The listing builds one solid part. Answer for the finished solid, in the listing's coordinates (mm). Face numbers are marked on the shaded views. A direction names the side the tool comes from. Give positions to 0.01 mm unless a question says otherwise; leave off trailing zeros. Order: outer loops, then holes, each group sorted by start corner. A loop starts at its lowest first (then second) coordinate and runs counter-clockwise, first axis right, second up. Notation, with made-up numbers: M -14.75,79.5 L 37.25,79.5 A30 ccw 37.25,101.5 Z; hole C 20,30.5 d11. An arc over 180 degrees is marked long. Answer as a JSON object with one key per item and string values. Group by question number.
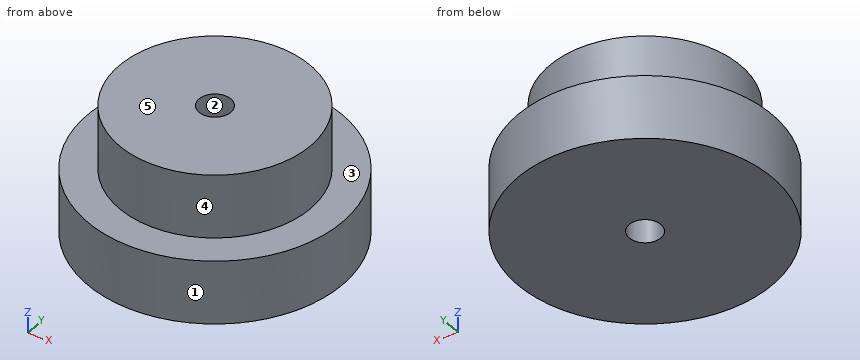
```python
from build123d import *

# Parameters (mm, degrees)
F0_R     = 10
F0_R_2   = 7.5
F1_DEPTH = 5
F2_R     = 7.5
F3_DEPTH = 5
F4_R     = 1.25
F5_DEPTH = 25.4


with BuildPart() as f1:
    # F0 (on Top) → F1 (new body)
    with BuildSketch(Plane.XY):
        Circle(F0_R)
        Circle(F0_R_2, mode=Mode.SUBTRACT)
        Circle(F0_R_2)
    extrude(amount=F1_DEPTH)

    # F2 (on face) → F3 (join)
    with BuildSketch(Plane.XY.offset(5)):
        Circle(F2_R)
    extrude(amount=F3_DEPTH)

    # F4 (on face) → F5 (cut)
    with BuildSketch(Plane.XY.offset(10)):
        Circle(F4_R)
    extrude(amount=-F5_DEPTH, mode=Mode.SUBTRACT)


solid = f1.part
```
Item 1: Determine the mould class of the marked faces 1, 2 and 3 for opening direction X: released by +X, released by -X, zero draft, split by the parting line, or undercut.
Item 2: Section A-A (y = 0) is taken. Determine the outline of the cut face in (x, z), and give its area (3 significant figures).
Item 3: Section D-D (y = -4) is taken. Determine the outline of the cut face in (x, z).
Item 4: Flat-ended cylindrical pins translate along their axes: P1, Ø1, axis at x = -7, z = 4, coming from the +Y side; P2, Ø3, axis at x = 3, z = 6, coming from the +Y side; P3, Ø4, axis at x = -7, z = 1.5, coming from the +Y side. Find the tip coordinate at first contact, or state that the pin passes through.
Item 5: Consider probe 1 along Y at (x, z) = (0, 2); probe 2 along Y at (x, z) = (0, 6.75); probe 3 along Z at (x, y) = (8.5, 1). Determine where each line is inside the solid, lowest interval first. Write a range as from..to.
Item 6: Section C-C (x = 6) is taken. Determine the outline of the cut face in (y, z).
Item 7: A tool of negligible diameter and unlimited length cuts with its end or side. For the marked faces 4 and 5, from which of +Z, -Z, +X, -X, +Y, -Y can it reach the whole face along a straight path? Write none if from no direction.
Values found:
{
 "1": {"face 1": "split by the parting line", "face 2": "undercut", "face 3": "zero draft"},
 "2": {"outline": "M -10,0 L -1.25,0 L -1.25,10 L -7.5,10 L -7.5,5 L -10,5 Z; M 1.25,0 L 10,0 L 10,5 L 7.5,5 L 7.5,10 L 1.25,10 Z", "area": "150 mm^2"},
 "3": {"outline": "M -9.17,0 L 9.17,0 L 9.17,5 L 6.34,5 L 6.34,10 L -6.34,10 L -6.34,5 L -9.17,5 Z"},
 "4": {"P1": "stops at y = 7.6", "P2": "stops at y = 9.82", "P3": "stops at y = 8.66"},
 "5": {"probe 1": "y = -10..-1.25, 1.25..10", "probe 2": "y = -7.5..-1.25, 1.25..7.5", "probe 3": "z = 0..5"},
 "6": {"outline": "M -8,0 L 8,0 L 8,5 L 4.5,5 L 4.5,10 L -4.5,10 L -4.5,5 L -8,5 Z"},
 "7": {"face 4": "+Z", "face 5": "+Z, +X, -X, +Y, -Y"}
}
